from build123d import *

# Parameters (mm, degrees)
BOSS_EXTRUDE1_DEPTH  = 12.572663867
SKETCH3_W            = 65.4
SKETCH3_H            = 30.4
BOSS_EXTRUDE2_DEPTH  = 43.572663867
FILLET1_R            = 9
SKETCH4_R            = 2.75
CUT_EXTRUDE1_DEPTH   = 20
CUT_EXTRUDE2_DEPTH   = 129
SKETCH6_R            = 6.7
CUT_EXTRUDE3_DEPTH   = 129
CUT_EXTRUDE6_DEPTH   = 63
SKETCH8_W            = 26.7
SKETCH8_H            = 1.112336133
BOSS_EXTRUDE3_DEPTH  = 4.2
BOSS_EXTRUDE4_DEPTH  = 41.15
SKETCH10_W           = 32.05
SKETCH10_H           = 5.146663352
BOSS_EXTRUDE5_DEPTH  = 4.2
BOSS_EXTRUDE6_DEPTH  = 23.35
CUT_EXTRUDE7_DEPTH   = 23.35
BOSS_EXTRUDE7_DEPTH  = 5
SKETCH15_W           = 32.05
SKETCH15_H           = 28.624452046
BOSS_EXTRUDE8_DEPTH  = 7.95
FILLET2_R            = 4
FILLET3_R            = 4
SKETCH16_R           = 2.2
CUT_EXTRUDE8_DEPTH   = 20
CUT_EXTRUDE9_DEPTH   = 41
BOSS_EXTRUDE9_DEPTH  = 5
SKETCH19_R           = 2.420474662
CUT_EXTRUDE10_DEPTH  = 5
BOSS_EXTRUDE10_START = -5
SKETCH20_R           = 2.420474662
SKETCH20_R_2         = 1.7
BOSS_EXTRUDE10_DEPTH = 5
SKETCH21_W           = 4
SKETCH21_H           = 10
CUT_EXTRUDE11_DEPTH  = 10


with BuildPart() as part:
    # Sketch2 → Boss-Extrude1 (new body)
    with BuildSketch(Plane.XZ):
        Polygon((-29.5, -30.2), (-32.5, -30.2), (-32.7, -30.2), (-32.7, -27), (-32.7, 0), (-32.7, 0.2), (32.5, 0.2), (32.7, 0.2), (32.900400589, -30.2), align=None)
    extrude(amount=BOSS_EXTRUDE1_DEPTH)

    # Sketch3 → Boss-Extrude2 (add)
    with BuildSketch(Plane(origin=(0, -12.572663867, 0), x_dir=(-1, 0, 0), z_dir=(0, -1, 0))):
        Polygon((-32.7, -5.2), (32.651437537, -5.2), (42.651437537, -5.2), (42.651437537, 30.2), (42.651437537, 35.2), (-32.900400589, 35.2), (-42.900400589, 35.2), (-42.900400589, 30.2), (-42.900400589, -5.2), align=None)
        with Locations((0, 15)):
            Rectangle(SKETCH3_W, SKETCH3_H, mode=Mode.SUBTRACT)
    extrude(amount=-BOSS_EXTRUDE2_DEPTH)

    # Fillet1
    fillet1_edges = [part.edges().sort_by_distance(p)[0] for p in [
        (42.900400589, 9.213668067, -35.2),
        (42.900400589, 9.213668067, 5.2),
    ]]
    fillet(fillet1_edges, radius=FILLET1_R)

    # Sketch4 → Cut-Extrude1 (cut)
    with BuildSketch(Plane(origin=(0, 31, 0), x_dir=(1, 0, 0), z_dir=(0, 1, 0))):
        with Locations(Location((-37.5, 23.5, 0), (0, 0, 270))):
            Circle(SKETCH4_R)
        with Locations(Location((-37.5, 6.5, 0), (0, 0, 270))):
            Circle(SKETCH4_R)
        with Locations(Location((37.5, 6.5, 0), (0, 0, 270))):
            Circle(SKETCH4_R)
        with Locations(Location((37.5, 23.5, 0), (0, 0, 270))):
            Circle(SKETCH4_R)
    extrude(amount=-CUT_EXTRUDE1_DEPTH, mode=Mode.SUBTRACT)

    # Sketch5 → Cut-Extrude2 (cut)
    with BuildSketch(Plane(origin=(42.900400589, 0, 0), x_dir=(0, 0, -1), z_dir=(1, 0, 0))):
        Polygon((6.5, 26), (3.8, 26), (3.8, 22), (10, 22), (10, 26), align=None)
        Polygon((26.2, 26), (23.5, 26), (20, 26), (20, 22), (26.2, 22), align=None)
    extrude(amount=-CUT_EXTRUDE2_DEPTH, mode=Mode.SUBTRACT)

    # Sketch6 → Cut-Extrude3 (cut)
    with BuildSketch(Plane.XZ.offset(12.572663867)):
        with Locations((19.5, -15)):
            Circle(SKETCH6_R)
    extrude(amount=-CUT_EXTRUDE3_DEPTH, mode=Mode.SUBTRACT)

    # Sketch7 → Cut-Extrude6 (cut)
    with BuildSketch(Plane(origin=(42.900400589, 0, 0), x_dir=(0, 0, -1), z_dir=(1, 0, 0))):
        Polygon((21.019628841, 3.612336133), (9.019628841, 3.612336133), (9.019628841, 9.612336133), (15.019628841, 9.612336133), (21.019628841, 9.612336133), align=None)
    extrude(amount=-CUT_EXTRUDE6_DEPTH, mode=Mode.SUBTRACT)

    # Sketch8 → Boss-Extrude3 (add)
    with BuildSketch(Plane.XY.offset(5.2)):
        with Locations((-29.301437537, 31.556168066)):
            Rectangle(SKETCH8_W, SKETCH8_H)
    extrude(amount=-BOSS_EXTRUDE3_DEPTH)

    # Sketch9 → Boss-Extrude4 (add)
    with BuildSketch(Plane.XY.offset(5.2)):
        Polygon((-15.951437537, 11.762336133), (-42.651437537, 11.762336133), (-42.651437537, 7.522211306), (-10.601437537, 7.522211306), (-10.601437537, 11.762336133), (-10.601437537, 31), (-15.601437537, 31), (-15.601437537, 11.762336133), align=None)
        Polygon((-42.651437537, 36.146663352), (-42.651437537, 32.462336133), (-15.601437537, 32.462336133), (-15.601437537, 32.112336133), (-15.601437537, 31), (-10.601437537, 31), (-10.601437537, 32.462336133), (-10.601437537, 36.146663352), align=None)
    extrude(amount=BOSS_EXTRUDE4_DEPTH)

    # Sketch10 → Boss-Extrude5 (add)
    with BuildSketch(Plane(origin=(0, 0, 5.2), x_dir=(-1, 0, 0), z_dir=(0, 0, -1))):
        with Locations((26.626437537, 33.573331676)):
            Rectangle(SKETCH10_W, SKETCH10_H)
    extrude(amount=BOSS_EXTRUDE5_DEPTH)

    # Sketch12 → Boss-Extrude6 (add)
    with BuildSketch(Plane(origin=(-10.601437537, 0, 0), x_dir=(0, 0, -1), z_dir=(1, 0, 0))):
        Polygon((-46.35, 21.834437329), (-46.35, 19.334437329), (-5.2, 19.334437329), (-5.2, 24.334437329), (-46.35, 24.334437329), align=None)
    extrude(amount=BOSS_EXTRUDE6_DEPTH)

    # Sketch13 → Cut-Extrude7 (cut)
    with BuildSketch(Plane(origin=(0, 24.334437329, 0), x_dir=(1, 0, 0), z_dir=(0, 1, 0))):
        Polygon((12.748562463, -5.2), (-10.601437537, -46.35), (12.748562463, -46.35), align=None)
    extrude(amount=-CUT_EXTRUDE7_DEPTH, mode=Mode.SUBTRACT)

    # Sketch14 → Boss-Extrude7 (add)
    with BuildSketch(Plane.ZY.offset(42.651437537)):
        Polygon((5.2, -12.572663867), (27.600666869, 7.522211306), (5.2, 7.522211306), align=None)
    extrude(amount=-BOSS_EXTRUDE7_DEPTH)

    # Sketch15 → Boss-Extrude8 (add)
    with BuildSketch(Plane.XY.offset(46.35)):
        with Locations((-26.626437537, 21.834437329)):
            Rectangle(SKETCH15_W, SKETCH15_H)
    extrude(amount=BOSS_EXTRUDE8_DEPTH)

    # Fillet2
    fillet2_edges = [part.edges().sort_by_distance(p)[0] for p in [
        (-10.601437537, 21.834437329, 54.3),
    ]]
    fillet(fillet2_edges, radius=FILLET2_R)

    # Fillet3
    fillet3_edges = [part.edges().sort_by_distance(p)[0] for p in [
        (-28.626437537, 7.522211306, 54.3),
        (-28.626437537, 36.146663352, 54.3),
        (-10.601437537, 36.146663352, 25.65),
        (-11.773010412, 36.146663352, 53.128427125),
        (-10.601437537, 7.522211306, 27.75),
        (-11.773010412, 7.522211306, 53.128427125),
    ]]
    fillet(fillet3_edges, radius=FILLET3_R)

    # Sketch16 → Cut-Extrude8 (cut)
    with BuildSketch(Plane.ZY.offset(42.651437537)):
        with Locations(Location((49.7, 27.062336133, 0), (0, 0, 270))):
            Circle(SKETCH16_R)
        with Locations(Location((49.7, 17.162336133, 0), (0, 0, 270))):
            Circle(SKETCH16_R)
        with Locations(Location((1.5, 27.062336133, 0), (0, 0, 270))):
            Circle(SKETCH16_R)
        with Locations(Location((1.5, 17.162336133, 0), (0, 0, 270))):
            Circle(SKETCH16_R)
    extrude(amount=-CUT_EXTRUDE8_DEPTH, mode=Mode.SUBTRACT)

    # Sketch17 → Cut-Extrude9 (cut)
    with BuildSketch(Plane.XY.offset(54.3)):
        Polygon((-33.651437537, 23.562336133), (-37.651437537, 23.562336133), (-37.651437537, 27.062336133), (-37.651437537, 30.562336133), (-33.651437537, 30.562336133), align=None)
        Polygon((-33.651437537, 20.106538525), (-37.651437537, 20.106538525), (-37.651437537, 16.606538525), (-37.651437537, 13.106538525), (-33.651437537, 13.106538525), align=None)
    extrude(amount=-CUT_EXTRUDE9_DEPTH, mode=Mode.SUBTRACT)

    # Sketch18 → Boss-Extrude9 (add)
    with BuildSketch(Plane.ZY.offset(42.651437537)):
        with BuildLine():
            Line((7.492385077, 44.529251739), (1, 36.146663352))
            Line((1, 36.146663352), (22.205551353, 36.146663352))
            Line((22.205551353, 36.146663352), (15.713166275, 44.529251739))
            ThreePointArc((15.713166275, 44.529251739), (11.602775676, 46.544776073), (7.492385077, 44.529251739))
        make_face()
        with BuildLine():
            ThreePointArc((11.602775676, 38.925245051), (9.891241629, 43.05725376), (14.023250338, 41.345719713))
            ThreePointArc((14.023250338, 41.345719713), (13.314309723, 39.634185666), (11.602775676, 38.925245051))
        make_face(mode=Mode.SUBTRACT)
    extrude(amount=-BOSS_EXTRUDE9_DEPTH)

    # Sketch19 → Cut-Extrude10 (cut)
    with BuildSketch(Plane.ZY.offset(42.651437537)):
        with Locations(Location((11.602775676, 2.878952554, 0), (0, 0, 270))):
            Circle(SKETCH19_R)
    extrude(amount=-CUT_EXTRUDE10_DEPTH, mode=Mode.SUBTRACT)

    # Sketch20 → Boss-Extrude10 (add)
    # profile 1 of 2: a face of its own
    with BuildSketch(Plane(origin=(-37.651437537, 0, 0), x_dir=(0, 0, -1), z_dir=(1, 0, 0)).offset(BOSS_EXTRUDE10_START)):
        with Locations((-11.602775676, 41.345719713)):
            Circle(SKETCH20_R)
        with Locations(Location((-11.602775676, 41.345719713, 0), (0, 0, 90))):
            Circle(SKETCH20_R_2, mode=Mode.SUBTRACT)
    # profile 2 of 2: a face of its own
    with BuildSketch(Plane(origin=(-37.651437537, 0, 0), x_dir=(0, 0, -1), z_dir=(1, 0, 0)).offset(BOSS_EXTRUDE10_START)):
        with Locations((-11.602775676, 2.878952554)):
            Circle(SKETCH20_R)
        with Locations(Location((-11.602775676, 2.878952554, 0), (0, 0, 90))):
            Circle(SKETCH20_R_2, mode=Mode.SUBTRACT)
    extrude(amount=BOSS_EXTRUDE10_DEPTH)

    # Sketch21 → Cut-Extrude11 (cut)
    with BuildSketch(Plane.XY.offset(54.3)):
        with Locations((-20.651437537, 21.834437329)):
            Rectangle(SKETCH21_W, SKETCH21_H)
    extrude(amount=-CUT_EXTRUDE11_DEPTH, mode=Mode.SUBTRACT)


solid = part.part
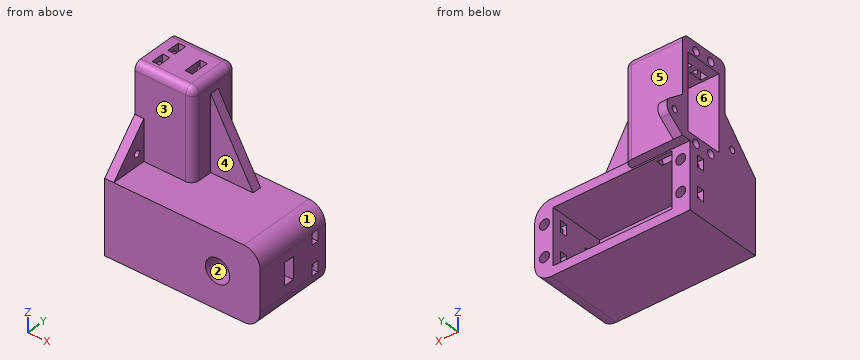
Geometry check sheet. Reference: the model listing, model coordinates, mm. Face numbers are marked on the shaded views. A direction names the side the tool comes from. Give positions to 0.01 mm unless a question says otherwise; leave off trailing zeros. Loops run counter-clockwise (first coordinate to the right, second up) from the corner with the lowest first, then second, coordinate; pieces in that order, holes last. Notation, with made-up numbers: (89, 49.5) -> (130, 49.5) arc R26 ccw to (130, 70.5) -> close; hole circle Ø8 at (9, 12). An arc over 180 degrees is marked (long way). Answer in a Markdown table with one row per item. Add a question column.
1) Cross-section at D-D on z = 38. Record the boundary of the cut face in (x, y).
2) Cross-section at A-A on z = -15. Record the boundary of the cut face in (x, y), and give its area (3 significant figures).
3) Cross-section at B-B on x = 19.5. Record the boundary of the cut face in (y, z), and give its area (3 significant figures).
4) Cross-section at C-C on x = -4. Record the boundary of the cut face in (y, z).
5) Gauge pin test, flat ends, axial feed: P1, Ø12, axis at x = -8.5, y = 37.5, coming from the +Z side; P2, Ø22, axis at y = -0.5, z = 17, coming from the +X side; P3, Ø2, axis at y = 37, z = -1, coming from the +X side; P4, Ø7, axis at x = 37.5, z = -6.5, coming from the +Y side. Record the tip position at first contact, or that the pin passes through.
6) Set-up check for the marked faces 4, 5 and 6: record each of +Z, -Z, +X, -X, +Y, -Y from which the full face is reachable in a straight line by a thin tool's end or side.
7) Material ranges on probe 1 along Z at (x, y) = (-10, 14); probe 2 along Y at (x, z) = (-29.5, 26.5); probe 3 along Z at (x, y) = (-37, 19), recorded low to high. Write a range as from..to.
8) Draft check along Z on the marked faces 1, 2 and 3. Enter one of: pulls with the +Z half, pulls with the -Z half, needs draft (parallel to the pull), parting line crosses it, or undercut.
Outcome:
| question | item | result |
|---|---|---|
| 1 | outline | (-42.65, 7.52) -> (-14.6, 7.52) arc R4 ccw to (-10.6, 11.52) -> (-10.6, 19.33) -> (-5.86, 19.33) -> (-5.86, 24.33) -> (-10.6, 24.33) -> (-10.6, 32.15) arc R4 ccw to (-14.6, 36.15) -> (-42.65, 36.15) -> (-42.65, 32.46) -> (-15.6, 32.46) -> (-15.6, 11.76) -> (-42.65, 11.76) -> close |
| 2 | outline | (-42.65, -12.57) -> (12.8, -12.57) -> (12.8, 0) -> (-32.7, 0) -> (-32.7, 31) -> (-42.65, 31) -> close; (26.2, -12.57) -> (42.9, -12.57) -> (42.9, 3.61) -> (32.7, 3.61) -> (32.7, 0) -> (26.2, 0) -> close; (32.7, 9.61) -> (42.9, 9.61) -> (42.9, 31) -> (32.7, 31) -> close |
| 2 | area | 1,470 mm^2 |
| 3 | outline | (-12.57, -35.2) -> (31, -35.2) -> (31, -30.2) -> (0, -30.2) -> (0, -21.7) -> (-12.57, -21.7) -> close; (-12.57, -8.3) -> (0, -8.3) -> (0, 0.2) -> (31, 0.2) -> (31, 5.2) -> (-12.57, 5.2) -> close |
| 3 | area | 649 mm^2 |
| 4 | outline | (-12.57, -35.2) -> (31, -35.2) -> (31, -30.2) -> (0, -30.2) -> (0, 0.2) -> (31, 0.2) -> (31, 5.2) -> (24.33, 5.2) -> (24.33, 34.72) -> (19.33, 34.72) -> (19.33, 5.2) -> (-12.57, 5.2) -> close |
| 5 | P1 | stops at z = 53.69 |
| 5 | P2 | stops at x = -10.73 |
| 5 | P3 | passes through |
| 5 | P4 | stops at y = 31 |
| 6 | face 4 | +Z, +X, -Y |
| 6 | face 5 | +Z, +X, +Y |
| 6 | face 6 | -X |
| 7 | probe 1 | z = -35.2..-30.2, 0.2..5.2 |
| 7 | probe 2 | y = 7.52..11.76, 32.46..36.15 |
| 7 | probe 3 | z = -35.2..-26.2, -20.8..-9.2, -3.8..0.29, 2.71..5.2 |
| 8 | face 1 | pulls with the +Z half |
| 8 | face 2 | undercut |
| 8 | face 3 | needs draft |
